Could you check a few things on this drawing? It's one solid part, dimensions in mm from its lowest x, y, z. A direction names the side the tool comes from. Coordinates: 2 decimals unless noted, no trailing zeros. Loops run counter-clockwise (first coordinate to the right, second up) from the corner with the lowest first, then second, coordinate; pieces in that order, holes last.
1) Will these pins go through, and if not, where does the flat tip stop? P1, Ø4, axis at x = 8.5, z = 34.5, coming from the -Y side; P2, Ø8, axis at x = 20, y = 20, coming from the +Z side; P3, Ø16, axis at x = 18, z = 10.5, coming from the +Y side.
2) Imagine slicing it at D-D on x = 11. Please give me the cut outline in (y, z), plus the area to 3 significant figures.
3) For the marked faces 1, 2 and 3, which set-ups out of +Z, -Z, +X, -X, +Y, -Y let a thin tool reach every point of the face, with its end or its side?
4) If I drill on line 1 along Y through (x, z) = (20, 0.35); line 2 along Y through (x, z) = (13, 34.5); line 3 along Y through (x, z) = (2, 27), over which ranges is the centre line in solid material (lowest first)?
5) Imagine slicing it at A-A on y = 35. Please give me the cut outline in (x, z), plus the area to 3 significant figures.
6) Imagine slicing it at C-C on z = 8. Please give me the cut outline in (x, y).
7) Imagine slicing it at B-B on x = 20. Please give me the cut outline in (y, z), plus the area to 3 significant figures.
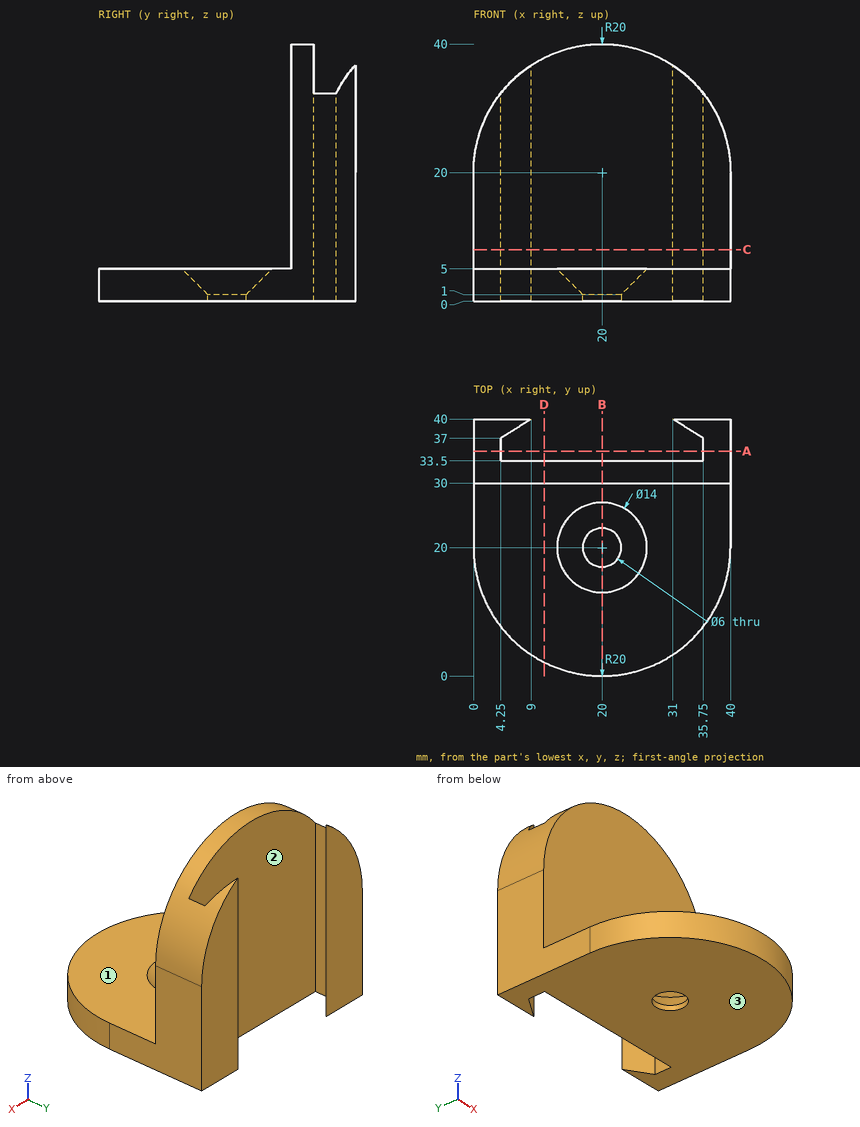
Filled in:
1. P1: stops at y = 30
1. P2: stops at z = 2
1. P3: stops at y = 33.5
2. outline: (2.14, 0) - (33.5, 0) - (33.5, 37.86) - (30, 37.86) - (30, 5) - (2.14, 5) - close
2. area: 272 mm2
3. face 1: +Z, +X, -X, -Y
3. face 2: +Z, -Z
3. face 3: -Z, +X, -X, +Y, -Y
4. line 1: y = 0 to 17, 23 to 33.5
4. line 2: y = 30 to 33.5
4. line 3: y = 30 to 40
5. outline: (0, 0) - (4.25, 0) - (4.25, 32.33) arc R20 ccw to (0, 20) - close; (35.75, 0) - (40, 0) - (40, 20) arc R20 ccw to (35.75, 32.33) - close
5. area: 241 mm2
6. outline: (0, 30) - (40, 30) - (40, 40) - (31, 40) - (35.75, 37) - (35.75, 33.5) - (4.25, 33.5) - (4.25, 37) - (9, 40) - (0, 40) - close
7. outline: (0, 0) - (17, 0) - (17, 1) - (13, 5) - (0, 5) - close; (23, 0) - (33.5, 0) - (33.5, 40) - (30, 40) - (30, 5) - (27, 5) - (23, 1) - close
7. area: 244 mm2
